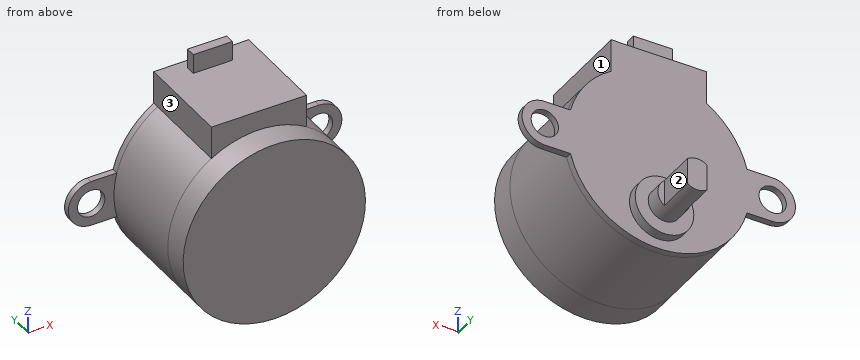
from build123d import *
from build123d.topology import SkipClean

# Parameters (mm, degrees)
SKETCH1_R           = 2.1
BOSS_EXTRUDE1_DEPTH = 1
BOSS_EXTRUDE2_START = -14
BOSS_EXTRUDE2_DEPTH = 14
BOSS_EXTRUDE3_START = 4
SKETCH3_R           = 14
BOSS_EXTRUDE3_DEPTH = 4
SKETCH4_R           = 4.5
BOSS_EXTRUDE4_DEPTH = 1.5
SKETCH5_R           = 2.5
BOSS_EXTRUDE5_DEPTH = 2.5
BOSS_EXTRUDE6_DEPTH = 6
SKETCH7_W           = 6
SKETCH7_H           = 1.5
BOSS_EXTRUDE7_DEPTH = 3


with BuildPart() as part:
    # Sketch1 → Boss-Extrude1 (new body)
    with BuildSketch(Plane(origin=(0, 0, 0), x_dir=(1, 0, 0), z_dir=(0, 1, 0))):
        with BuildLine():
            Line((-17.5, 3.5), (-13.555441712, 3.5))
            ThreePointArc((-13.555441712, 3.5), (0, 14), (13.555441712, 3.5))
            Line((13.555441712, 3.5), (17.5, 3.5))
            ThreePointArc((17.5, 3.5), (21, 0), (17.5, -3.5))
            Line((17.5, -3.5), (13.555441712, -3.5))
            ThreePointArc((13.555441712, -3.5), (11.250406053, -8.332368429), (7.3, -11.94612908))
            Line((7.3, -11.94612908), (7.3, -17))
            Line((7.3, -17), (-7.3, -17))
            Line((-7.3, -17), (-7.3, -11.94612908))
            ThreePointArc((-7.3, -11.94612908), (-11.250406053, -8.332368429), (-13.555441712, -3.5))
            Line((-13.555441712, -3.5), (-17.5, -3.5))
            ThreePointArc((-17.5, -3.5), (-21, 0), (-17.5, 3.5))
        make_face()
        with Locations(Location((-17.5, 0, 0), (0, 0, 270))):
            Circle(SKETCH1_R, mode=Mode.SUBTRACT)
        with Locations(Location((17.5, 0, 0), (0, 0, 270))):
            Circle(SKETCH1_R, mode=Mode.SUBTRACT)
    extrude(amount=BOSS_EXTRUDE1_DEPTH)

    # Sketch2 → Boss-Extrude2 (add)
    with SkipClean():  # the faces are left unmerged after this step: merging them gives an invalid solid
        with BuildSketch(Plane(origin=(0, 0, 0), x_dir=(1, 0, 0), z_dir=(0, 1, 0)).offset(BOSS_EXTRUDE2_START)):
            with BuildLine():
                Line((-7.3, -17), (7.3, -17))
                Line((7.3, -17), (7.3, -11.94612908))
                ThreePointArc((7.3, -11.94612908), (0, 14), (-7.3, -11.94612908))
                Line((-7.3, -11.94612908), (-7.3, -17))
            make_face()
        extrude(amount=BOSS_EXTRUDE2_DEPTH)

    # Sketch3 → Boss-Extrude3 (add)
    with SkipClean():  # the faces are left unmerged after this step: merging them gives an invalid solid
        with BuildSketch(Plane.XZ.offset(14).offset(BOSS_EXTRUDE3_START)):
            with Locations(Location((0, 0, 0), (0, 0, 270))):
                Circle(SKETCH3_R)
        extrude(amount=-BOSS_EXTRUDE3_DEPTH)

    # Sketch4 → Boss-Extrude4 (add)
    with SkipClean():  # the faces are left unmerged after this step: merging them gives an invalid solid
        with BuildSketch(Plane(origin=(0, 1, 0), x_dir=(1, 0, 0), z_dir=(0, 1, 0))):
            with Locations(Location((0, 8, 0), (0, 0, 270))):
                Circle(SKETCH4_R)
        extrude(amount=BOSS_EXTRUDE4_DEPTH)

    # Sketch5 → Boss-Extrude5 (add)
    with SkipClean():  # the faces are left unmerged after this step: merging them gives an invalid solid
        with BuildSketch(Plane(origin=(0, 2.5, 0), x_dir=(1, 0, 0), z_dir=(0, 1, 0))):
            with Locations(Location((0, 8, 0), (0, 0, 270))):
                Circle(SKETCH5_R)
        extrude(amount=BOSS_EXTRUDE5_DEPTH)

    # Sketch6 → Boss-Extrude6 (add)
    with SkipClean():  # the faces are left unmerged after this step: merging them gives an invalid solid
        with BuildSketch(Plane(origin=(0, 5, 0), x_dir=(1, 0, 0), z_dir=(0, 1, 0))):
            with BuildLine():
                ThreePointArc((-1.5, 6), (0, 5.5), (1.5, 6))
                Line((1.5, 6), (1.5, 10))
                ThreePointArc((1.5, 10), (0, 10.5), (-1.5, 10))
                Line((-1.5, 10), (-1.5, 6))
            make_face()
        extrude(amount=BOSS_EXTRUDE6_DEPTH)

    # Sketch7 → Boss-Extrude7 (add)
    with SkipClean():  # the faces are left unmerged after this step: merging them gives an invalid solid
        with BuildSketch(Plane.XY.offset(17)):
            with Locations((0, -1.25)):
                Rectangle(SKETCH7_W, SKETCH7_H)
        extrude(amount=BOSS_EXTRUDE7_DEPTH)


solid = part.part
Verification items for the finished model (mm, model axes). Face numbers are marked on the shaded views. A direction names the side the tool comes from. Coordinates: 2 decimals unless noted, no trailing zeros. Loops run counter-clockwise (first coordinate to the right, second up) from the corner with the lowest first, then second, coordinate; pieces in that order, holes last. Notation, with made-up numbers: (-34, 52) -> (-14, 52) arc R25 ccw to (-14, 73) -> close; hole circle Ø7 at (-37, 6). An arc over 180 degrees is marked (long way). Answer as a JSON object with one key per item and string values. Group by question number.
Item 1: Sectioned sample at C-C on x = 0. Record the boundary of the cut face in (y, z).
Item 2: Depth check by flat-ended pin: pin 1 (5.5 mm diameter, centred on x = 17.5, z = 0, fed in from +Y); pin 2 (1.5 mm diameter, centred on x = 5, y = 3.5, fed in from -Z); pin 3 (0.5 mm diameter, centred on x = 2, z = -8, fed in from +Y); pin 4 (10 mm diameter, centred on y = -5.5, z = 8, fed in from +X). Enter the tip coordinate at first touch or a pass-through.
Item 3: Sectioned sample at A-A on z = 0. Record the boundary of the cut face in (x, y).
Item 4: Sectioned sample at D-D on z = -8. Record the boundary of the cut face in (x, y).
Item 5: Tool access check on the marked faces 1, 2 and 3. Record the directions out of +Z, -Z, +X, -X, +Y, -Y that give a thin tool (end or side, any length) a straight path to the whole face; none if there is none.
Item 6: Sectioned sample at B-B on y = -1. Record the boundary of the cut face in (x, z), plus the area to 3 significant figures.
Item 7: Scan lines: probe 1 along X at (y, z) = (0.75, 0); probe 2 along Y at (x, z) = (15.5, 1); probe 3 along Y at (x, z) = (5.5, 14). Record each from-to range of solid material in increasing order.
Evaluation:
{
 "1": {"outline": "(-18, -14) -> (1, -14) -> (1, -12.5) -> (2.5, -12.5) -> (2.5, -10.5) -> (11, -10.5) -> (11, -5.5) -> (2.5, -5.5) -> (2.5, -3.5) -> (1, -3.5) -> (1, 17) -> (-0.5, 17) -> (-0.5, 20) -> (-2, 20) -> (-2, 17) -> (-14, 17) -> (-14, 14) -> (-18, 14) -> close"},
 "2": {"pin 1": "stops at y = 1", "pin 2": "passes through", "pin 3": "stops at y = 5", "pin 4": "stops at x = 13.67"},
 "3": {"outline": "(-21, 0) -> (-19.6, 0) -> (-19.6, 1) -> (-21, 1) -> close; (-15.4, 0) -> (-14, 0) -> (-14, -18) -> (14, -18) -> (14, 0) -> (15.4, 0) -> (15.4, 1) -> (-15.4, 1) -> close; (19.6, 0) -> (21, 0) -> (21, 1) -> (19.6, 1) -> close"},
 "4": {"outline": "(-11.49, -18) -> (11.49, -18) -> (11.49, 1) -> (4.5, 1) -> (4.5, 2.5) -> (2.5, 2.5) -> (2.5, 5) -> (1.5, 5) -> (1.5, 11) -> (-1.5, 11) -> (-1.5, 5) -> (-2.5, 5) -> (-2.5, 2.5) -> (-4.5, 2.5) -> (-4.5, 1) -> (-11.49, 1) -> close"},
 "5": {"face 1": "+Z, +X, +Y, -Y", "face 2": "+Z, -Z, +X, +Y", "face 3": "+Z, -X, +Y, -Y"},
 "6": {"outline": "(-7.3, 11.95) arc R14 ccw (long way) to (7.3, 11.95) -> (7.3, 17) -> (3, 17) -> (3, 20) -> (-3, 20) -> (-3, 17) -> (-7.3, 17) -> close", "area": "687 mm²"},
 "7": {"probe 1": "x = -21 to -19.6, -15.4 to 15.4, 19.6 to 21", "probe 2": "y = 0 to 1", "probe 3": "y = -14 to 1"}
}
